from build123d import *

# Parameters (mm, degrees)
SKETCH1_R           = 6.05
SKETCH1_R_2         = 9.05
BOSS_EXTRUDE1_DEPTH = 5
CUT_EXTRUDE1_START  = -2
CUT_EXTRUDE1_DEPTH  = 2


with BuildPart() as part:
    # Sketch1 → Boss-Extrude1 (new body)
    with BuildSketch(Plane.XY):
        with BuildLine():
            Line((-17.428425058, 4.5), (-24.206145914, -21.75))
            ThreePointArc((-24.206145914, -21.75), (-24.304944461, -33.854030643), (-18.705990528, -44.585714286))
            ThreePointArc((-18.705990528, -44.585714286), (-16.188386739, -51.22), (-18.705990528, -57.854285714))
            ThreePointArc((-18.705990528, -57.854285714), (-14.737892988, -94.633922608), (21.5, -87.197350822))
            Line((21.5, -87.197350822), (35.277938888, -63.977350822))
            ThreePointArc((35.277938888, -63.977350822), (38.71637128, -52.973450833), (36.851550967, -41.59667284))
            Line((36.851550967, -41.59667284), (16.613000697, 6.928795555))
            ThreePointArc((16.613000697, 6.928795555), (-1.281011782, 17.954359048), (-17.428425058, 4.5))
        make_face()
        with Locations((0, -28)):
            Circle(SKETCH1_R, mode=Mode.SUBTRACT)
        with Locations((13.777938888, -51.22)):
            Circle(SKETCH1_R_2, mode=Mode.SUBTRACT)
        with Locations((0, -74.44)):
            Circle(SKETCH1_R_2, mode=Mode.SUBTRACT)
    extrude(amount=BOSS_EXTRUDE1_DEPTH)

    # Sketch2 → Cut-Extrude1 (cut)
    with BuildSketch(Plane.XY.offset(5).offset(CUT_EXTRUDE1_START)):
        with BuildLine():
            Line((16.613000697, 6.928795555), (36.851550967, -41.59667284))
            ThreePointArc((36.851550967, -41.59667284), (38.71637128, -52.973450833), (35.277938888, -63.977350822))
            Line((35.277938888, -63.977350822), (21.5, -87.197350822))
            ThreePointArc((21.5, -87.197350822), (-14.737892988, -94.633922608), (-18.705990528, -57.854285714))
            ThreePointArc((-18.705990528, -57.854285714), (-16.188386739, -51.22), (-18.705990528, -44.585714286))
            ThreePointArc((-18.705990528, -44.585714286), (-24.304944461, -33.854030643), (-24.206145914, -21.75))
            Line((-24.206145914, -21.75), (-17.428425058, 4.5))
            ThreePointArc((-17.428425058, 4.5), (-1.281011782, 17.954359048), (16.613000697, 6.928795555))
        make_face()
        with BuildLine():
            Line((9.468285508, 9.39955156), (5.467787499, 2.470485754))
            ThreePointArc((5.467787499, 2.470485754), (3, 5.196152423), (-0.594390327, 5.970485754))
            Line((-0.594390327, 5.970485754), (3.406107682, 12.89955156))
            ThreePointArc((3.406107682, 12.89955156), (3.46289335, 14.794014563), (1.913207856, 15.885201783))
            ThreePointArc((1.913207856, 15.885201783), (-9.022746373, 13.213252737), (-15.491933385, 4))
            Line((-15.491933385, 4), (-22.269654241, -22.25))
            ThreePointArc((-22.269654241, -22.25), (-20.946970822, -37.498653241), (-10.347792006, -48.540769231))
            ThreePointArc((-10.347792006, -48.540769231), (-8.697504007, -51.22), (-10.347792006, -53.899230769))
            ThreePointArc((-10.347792006, -53.899230769), (-16.813726675, -90.133903125), (19.78, -86.176762756))
            Line((19.78, -86.176762756), (21.416047429, -83.419527323))
            ThreePointArc((21.416047429, -83.419527323), (22.868749584, -79.189380689), (22.517294907, -74.730573258))
            ThreePointArc((22.517294907, -74.730573258), (22.927957655, -72.188598464), (25.15802624, -70.901324657))
            ThreePointArc((25.15802624, -70.901324657), (28.527716294, -69.789192601), (31.009004018, -67.252490018))
            Line((31.009004018, -67.252490018), (33.557938888, -62.956762756))
            ThreePointArc((33.557938888, -62.956762756), (36.721296689, -52.833174766), (35.005662001, -42.366539013))
            Line((35.005662001, -42.366539013), (24.369440107, -16.864334436))
            ThreePointArc((24.369440107, -16.864334436), (22.811532345, -15.020784633), (20.47666212, -14.409120101))
            ThreePointArc((20.47666212, -14.409120101), (17.701744194, -12.866781789), (17.865596008, -9.696272437))
            ThreePointArc((17.865596008, -9.696272437), (19.084800596, -6.438585473), (18.585469893, -2.996252973))
            Line((18.585469893, -2.996252973), (14.76711173, 6.158929383))
            ThreePointArc((14.76711173, 6.158929383), (13.890682857, 7.940335621), (12.800384361, 9.599487498))
            ThreePointArc((12.800384361, 9.599487498), (11.080545761, 10.395960893), (9.468285508, 9.39955156))
        make_face(mode=Mode.SUBTRACT)
    extrude(amount=CUT_EXTRUDE1_DEPTH, mode=Mode.SUBTRACT)


solid = part.part
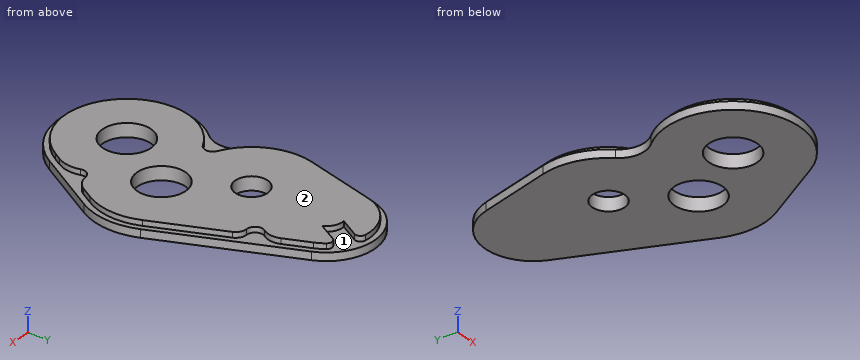
Input: part model. Units: mm. Frame: model coordinates. Face numbers are marked on the shaded views. A direction names the side the tool comes from. Give positions to 0.01 mm unless a question says otherwise; leave off trailing zeros. Write each loop counter-clockwise with the first axis right and the second up, starting at its lowest first coordinate (ties: lowest second). Pieces come first, ordered by that corner, then holes. Notation, with made-up numbers: (-38, 64.25) -> (-12, 64.25) arc R24 cw to (-12, 98.25) -> close; hole circle Ø11 at (10.25, -9.5). An arc over 180 degrees is marked (long way). Use one line per item in the form item = value. Start each with the question number.
1) Section query C-C on x = -11.5. Return the cut outline in (y, z).
2) Section query D-D on y = -7. Return the cut outline in (x, z), then the cut area to 3 significant figures.
3) Section query B-B on z = 2. Return the cut outline in (x, y).
4) Ray query, probe 1 along Y at (x, z) = (0, 2.45); probe 2 along Y at (x, z) = (0, 3.15); probe 3 along Y at (x, z) = (1.5, 4.4). Return the intervals inside material, ascending. Write a range as from..to.
5) Pin query (flat end, axial travel): pin 1 (2 mm diameter, centred on y = -14, z = 4.5, fed in from +X); pin 2 (1 mm diameter, centred on y = -50.5, z = 4.5, fed in from +X); pin 3 (2 mm diameter, centred on x = -7, z = 1.5, fed in from -Y). Return the tip coordinate at first contact, or that it passes through.
6) Section query A-A on y = -51.22. Return the cut outline in (x, z), then the cut area to 3 significant figures.
7) Set-up query: the marked faces 1 and 2. Return all of +Z, -Z, +X, -X, +Y, -Y with unobstructed straight access to the full face (end or side cutting, diameter ignored); none if empty.
Outcome:
q1.outline = (-96.64, 0) -> (13.85, 0) -> (13.85, 3) -> (11.12, 3) -> (11.12, 5) -> (-47.92, 5) -> (-47.92, 3) -> (-54.52, 3) -> (-54.52, 5) -> (-94.36, 5) -> (-94.36, 3) -> (-96.64, 3) -> close
q2.outline = (-20.4, 0) -> (22.42, 0) -> (22.42, 3) -> (19, 3) -> (19, 5) -> (-18.33, 5) -> (-18.33, 3) -> (-20.4, 3) -> close
q2.area = 203 mm^2
q3.outline = (-24.21, -21.75) arc R25 ccw to (-18.71, -44.59) arc R10 cw to (-18.71, -57.85) arc R25 ccw (long way) to (21.5, -87.2) -> (35.28, -63.98) arc R25 ccw to (36.85, -41.6) -> (16.61, 6.93) arc R18 ccw to (-17.43, 4.5) -> close; hole circle Ø18.1 at (0, -74.44); hole circle Ø12.1 at (0, -28); hole circle Ø18.1 at (13.78, -51.22)
q4.probe_1 = -99.44..-83.49, -65.39..-34.05, -21.95..18
q4.probe_2 = -97.44..-83.49, -65.39..-34.05, -21.95..6, 7..16
q4.probe_3 = -97.39..-83.36, -65.52..-33.86, -22.14..5.81, 9.6..15.93
q5.pin_1 = 22.78
q5.pin_2 = 36.78
q5.pin_3 = -98.71
q6.outline = (-16.19, 0) -> (4.73, 0) -> (4.73, 5) -> (-8.7, 5) -> (-8.7, 3) -> (-16.19, 3) -> close; (22.83, 0) -> (38.78, 0) -> (38.78, 3) -> (36.78, 3) -> (36.78, 5) -> (22.83, 5) -> close
q6.area = 165 mm^2
q7.face_1 = +Z
q7.face_2 = +Z, +X, -X, +Y, -Y
